Model file for the job. Use its own axes, mm. Face numbers are marked on the shaded views. A direction names the side the tool comes from. Coordinates: 2 decimals unless noted, no trailing zeros. Loops run counter-clockwise (first coordinate to the right, second up) from the corner with the lowest first, then second, coordinate; pieces in that order, holes last.
from build123d import *

# Parameters (mm, degrees)
F0_R     = 3.35
F1_DEPTH = 1.8
F2_R     = 5
F3_DEPTH = 4.8
F4_R     = 0.5
F5_SIZE  = 0.5


with BuildPart() as f1:
    # F0 (on Top) → F1 (new body)
    with BuildSketch(Plane.XY):
        with BuildLine():
            Line((-5.5425625842, -9.6), (5.5425625842, -9.6))
            ThreePointArc((5.5425625842, -9.6), (7.7462161651, -4.4722799881), (11.0851251684, 0))
            Line((11.0851251684, 0), (5.5425625842, 9.6))
            Line((5.5425625842, 9.6), (-5.5425625842, 9.6))
            Line((-5.5425625842, 9.6), (-11.0851251684, 0))
            ThreePointArc((-11.0851251684, 0), (-7.745470711, -4.4718496), (-5.5425625842, -9.6))
        make_face()
        Polygon((7.3900834456, 0), (3.6950417228, -6.4), (-3.6950417228, -6.4), (-7.3900834456, 0), (-3.6950417228, 6.4), (3.6950417228, 6.4), align=None, mode=Mode.SUBTRACT)
        Polygon((-3.6950417228, -6.4), (3.6950417228, -6.4), (7.3900834456, 0), (3.6950417228, 6.4), (-3.6950417228, 6.4), (-7.3900834456, 0), align=None)
        Circle(F0_R, mode=Mode.SUBTRACT)
    extrude(amount=F1_DEPTH)

    # F2
    f2_edges = [f1.edges().sort_by_distance(p)[0] for p in [
        (-11.085125, 0, 0.9),
        (-5.542563, 9.6, 0.9),
        (5.542563, 9.6, 0.9),
        (11.085125, 0, 0.9),
    ]]
    fillet(f2_edges, radius=F2_R)

    # F0 (on Top) → F3 (join)
    with BuildSketch(Plane.XY):
        Circle(F0_R)
    extrude(amount=F3_DEPTH)

    # F4
    f4_edges = [f1.edges().sort_by_distance(p)[0] for p in [
        (-3.35, 0, 4.8),
    ]]
    fillet(f4_edges, radius=F4_R)

    # F5
    f5_edges = [f1.edges().sort_by_distance(p)[0] for p in [
        (-5.155811, 8.930127, 0),
    ]]
    chamfer(f5_edges, length=F5_SIZE)


solid = f1.part
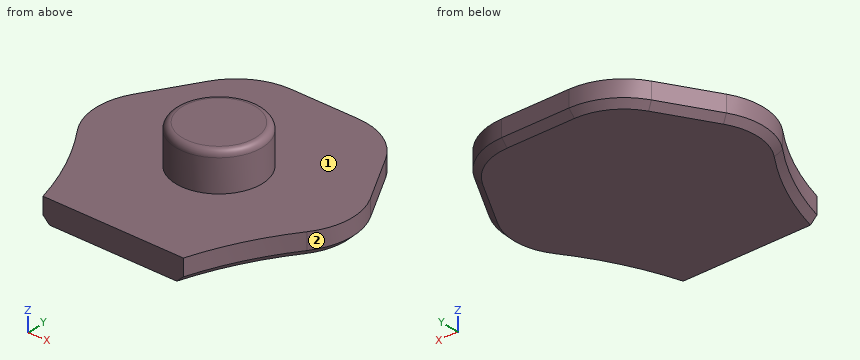
Q1. Flat gauge pins, fed straight in: P1, Ø6, axis at x = -6.5, y = -2.5, coming from the +Z side; P2, Ø1.5, axis at y = -2.5, z = 4, coming from the -X side; P3, Ø2, axis at y = 3, z = 1.5, coming from the +X side. Where does each tip first touch, or does it go through?
Answers:
P1: stops at z = 1.8
P2: stops at x = -2.86
P3: stops at x = 9.79
Q2. Which spindle directions (+Z, -Z, +X, -X, +Y, -Y) get a long thin tool onto all of the face, cutting with end or side? Do the marked faces 1 and 2. Say none if no direction does.
Answers:
face 1: +Z
face 2: +Z, -Z, +X
Q3. Slice it at A-A (x = 0). List the corners of the cut face in (y, z), and give its area (3 significant figures).
Answers:
outline: (-9.6, 0) - (9.1, 0) - (9.6, 0.5) - (9.6, 1.8) - (3.35, 1.8) - (3.35, 4.3) arc R0.5 ccw to (2.85, 4.8) - (-2.85, 4.8) arc R0.5 ccw to (-3.35, 4.3) - (-3.35, 1.8) - (-9.6, 1.8) - close
area: 54.4 mm2
Q4. Slice it at C-C (z = 2.4). List the corners of the cut face in (x, y).
Answers:
outline: circle Ø6.7 at (0, 0)
Q5. Slice it at B-B (y = 3.75). List the corners of the cut face in (x, z), and give its area (3 significant figures).
Answers:
outline: (-8.92, 0.5) - (-8.34, 0) - (8.34, 0) - (8.92, 0.5) - (8.92, 1.8) - (-8.92, 1.8) - close
area: 31.8 mm2
Q6. Drill centre lines: line 1 (Z direction, x = -6.75, y = 3.75); line 2 (X direction, y = 2, z = 4.45); line 3 (Y direction, x = -1.25, z = 3.3). Where is each one in solid material? Low to high.
Answers:
line 1: z = 0 to 1.8
line 2: x = -2.66 to 2.66
line 3: y = -3.11 to 3.11
